Input: part model. Units: mm. Frame: model coordinates. Round coordinates to 2 decimals unless told otherwise and drop trailing zeros. Loops run counter-clockwise (first coordinate to the right, second up) from the corner with the lowest first, then second, coordinate; pieces in that order, holes last. Notation, with made-up numbers: M -11.5,46 L -7.5,46 A18 cw -7.5,76 Z; hole C -22.5,83.25 d7. An arc over 180 degrees is marked long. Put each result on its own line as item: value. Start each with the question number.
1) Section C-C on z = -13. Output: boundary loops of the cut face in (x, y), plus the area to 3 significant figures.
2) Section D-D on z = 12.5. Output: boundary loops of the cut face in (x, y).
3) Section B-B on x = 10.75. Output: boundary loops of the cut face in (y, z).
4) Pin query (flat end, axial travel): pin 1 (5 mm diameter, centred on x = 3.5, z = 1.5, fed in from -Y); pin 2 (1.5 mm diameter, centred on y = 0.5, z = 9, fed in from -X). Return the tip coordinate at first contact, or that it passes through.
5) Line query: probe 1 along X at (y, z) = (2.1, 22); probe 2 along Z at (x, y) = (1.25, 2.35); probe 3 along Z at (x, y) = (-0.5, 2.2). Output: solid intervals per line, ascending.
6) Section A-A on z = -5.5. Output: boundary loops of the cut face in (x, y), plus the area to 3 significant figures.
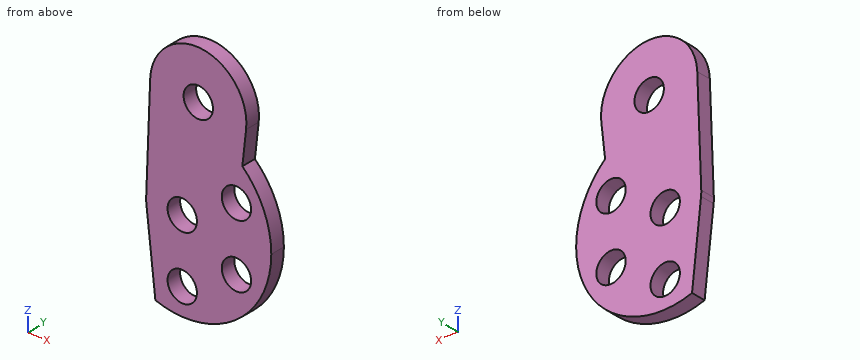
from build123d import *

# Parameters (mm, degrees)
SKETCH_1_R          = 7.5
SKETCH_1_R_2        = 3.05
EXTRUDE_1_DEPTH     = 3
SKETCH_2_R          = 3.05
EXTRUDE_2_DEPTH     = 3
SKETCH_3_R          = 3.05
CUT_EXTRUDE_1_DEPTH = 37.865769394


with BuildPart() as part:
    # 草图1 → 凸台-拉伸1 (new body)
    # profile 1 of 2: a face of its own
    with BuildSketch(Plane(origin=(0, 0, 0), x_dir=(1, 0, 0), z_dir=(0, 1, 0))):
        Circle(SKETCH_1_R)
    # profile 2 of 2: a face of its own
    with BuildSketch(Plane(origin=(0, 0, 0), x_dir=(1, 0, 0), z_dir=(0, 1, 0))):
        with BuildLine():
            ThreePointArc((18.5, 0), (10.931866676, 14.924620296), (-5.58046389, 17.638265866))
            Line((-5.58046389, 17.638265866), (-7.453841227, 0.830813432))
            ThreePointArc((-7.453841227, 0.830813432), (0.41604735, 7.488451416), (7.5, 0))
            ThreePointArc((7.5, 0), (4.104533282, -6.277165486), (-3.007415076, -6.870622574))
            Line((-3.007415076, -6.870622574), (12.484954374, -13.651956427))
            ThreePointArc((12.484954374, -13.651956427), (16.9295844, -7.45916698), (18.5, 0))
        make_face()
        with Locations(Location((11.258330249, -6.5, 0), (0, 0, 270))):
            Circle(SKETCH_1_R_2, mode=Mode.SUBTRACT)
        with Locations(Location((11.258330249, 6.5, 0), (0, 0, 270))):
            Circle(SKETCH_1_R_2, mode=Mode.SUBTRACT)
        with Locations(Location((0, 13, 0), (0, 0, 270))):
            Circle(SKETCH_1_R_2, mode=Mode.SUBTRACT)
    extrude(amount=EXTRUDE_1_DEPTH)

    # 草图2 → 凸台-拉伸2 (add, through all)
    with BuildSketch(Plane(origin=(0, 3, 0), x_dir=(1, 0, 0), z_dir=(0, 1, 0))):
        with BuildLine():
            ThreePointArc((-3.007415076, -6.870622574), (-6.197847944, -4.223349483), (-7.49455821, -0.285652289))
            Line((-7.49455821, -0.285652289), (-6.662072489, -22.1272861))
            ThreePointArc((-6.662072489, -22.1272861), (4.07930362, -31.718354527), (13.268273691, -20.6310382))
            Line((13.268273691, -20.6310382), (12.484954374, -13.651956427))
            Line((12.484954374, -13.651956427), (-3.007415076, -6.870622574))
        make_face()
        with Locations(Location((3.330671791, -21.746416381, 0), (0, 0, 270))):
            Circle(SKETCH_2_R, mode=Mode.SUBTRACT)
    extrude(amount=-EXTRUDE_2_DEPTH)

    # 草图3 → 切除-拉伸1 (cut, through all)
    with BuildSketch(Plane(origin=(0, 3, 0), x_dir=(1, 0, 0), z_dir=(0, 1, 0))):
        with Locations(Location((0, 0, 0), (0, 0, 270))):
            Circle(SKETCH_3_R)
    extrude(amount=-CUT_EXTRUDE_1_DEPTH, mode=Mode.SUBTRACT)


solid = part.part
Geometry results:
1. outline: M -6.1,0 L -3.05,0 L -3.05,3 L -6.1,3 Z; M 3.05,0 L 13.16,0 L 13.16,3 L 3.05,3 Z
1. area: 39.5 mm²
2. outline: M -7.03,0 L 13.64,0 L 13.64,3 L -7.03,3 Z
3. outline: M 0,-15.06 L 3,-15.06 L 3,-9.51 L 0,-9.51 Z; M 0,-3.49 L 3,-3.49 L 3,3.49 L 0,3.49 Z; M 0,9.51 L 3,9.51 L 3,28.45 L 0,28.45 Z
4. pin 1: stops at y = 0
4. pin 2: stops at x = -7.19
5. probe 1: x = -6.67 to 0.29, 6.37 to 13.33
5. probe 2: z = -18.46 to -15.78, -10.22 to -2.78, 2.78 to 19.52, 23.98 to 31.53
5. probe 3: z = -18.49 to -16.01, -9.99 to -3.01, 3.01 to 30.98
6. outline: M -6.93,0 L 8.38,0 L 8.38,3 L -6.93,3 Z; M 14.14,0 L 17.66,0 L 17.66,3 L 14.14,3 Z
6. area: 56.5 mm²
